Source: CAD feature listing. Evaluate the final solid. Frame: model axes, mm. Round coordinates to 2 decimals unless told otherwise and drop trailing zeros. Order: outer loops, then holes, each group sorted by start corner. A loop starts at its lowest first (then second) coordinate and runs counter-clockwise, first axis right, second up. Notation, with made-up numbers: M 14.25,58.5 L 19.25,58.5 A32 cw 19.25,92.5 Z; hole C 9,69 d2. An arc over 180 degrees is marked long. Answer in a Markdown table with one row per item. Add a question column.
```python
from build123d import *

# Parameters (mm, degrees)
F0_W     = 20
F0_H     = 20
F1_DEPTH = 25
F3_DEPTH = 20
F4_DEPTH = 30
F5_DEPTH = 25


with BuildPart() as f1:
    # F0 (on Front) → F1 (new body, symmetric)
    with BuildSketch(Plane.XZ):
        Rectangle(F0_W, F0_H)
        Polygon((20, -10), (10, 10), (10, -10), align=None)
        Polygon((20, 10), (10, 10), (20, -10), align=None)
        Polygon((-10, -10), (-10, 10), (-20, -10), align=None)
        Polygon((-20, -10), (-10, 10), (-20, 10), align=None)
    extrude(amount=F1_DEPTH, both=True)

    # F2 (on Right) → F3 (join, symmetric)
    with BuildSketch(Plane.YZ):
        Polygon((-25, -10), (-25, 0), (-25, 10), (-27.5, -10), align=None)
        Polygon((25, 10), (25, 0), (25, -10), (27.5, -10), align=None)
    extrude(amount=F3_DEPTH, both=True)

    # F0 (on Front) → F4 (cut, symmetric)
    with BuildSketch(Plane.XZ):
        Polygon((20, 10), (10, 10), (20, -10), align=None)
        Polygon((-20, -10), (-10, 10), (-20, 10), align=None)
    extrude(amount=F4_DEPTH, both=True, mode=Mode.SUBTRACT)

    # F2 (on Right) → F5 (cut, symmetric)
    with BuildSketch(Plane.YZ):
        Polygon((12.5, 9), (12.5, 10), (12, 10), align=None)
        Polygon((12.5, 9), (13, 10), (12.5, 10), align=None)
        Polygon((-12.5, 10), (-13, 10), (-12.5, 9), align=None)
        Polygon((-12, 10), (-12.5, 10), (-12.5, 9), align=None)
    extrude(amount=F5_DEPTH, both=True, mode=Mode.SUBTRACT)


solid = f1.part
```
(1) Draft query along Z for faces 1 (the face through (0, 0, 10)), 2 (the face through (0, 0, -10)). Return one class per face: +Z half, -Z half, draft (parallel to the pull), parting line (faces both ways), or undercut.
(2) Cut plane B-B (z = 6). Return loops of the section in (x, y), and give its area (3 significant figures).
(3) Cut plane A-A (x = 2). Return loops of the section in (y, z).
(4) Line query: line 1 (Z direction, x = 16, y = -14); line 2 (X direction, y = -2, z = -5.75) (3 decimals); line 3 (X direction, y = 19, z = 1.75) (3 decimals). Output: solid intervals per line, ascending. Write a range as from..to.
(5) Cut plane C-C (y = 1). Return loops of the section in (x, z), and give its area (3 significant figures).
(6) Pin query (flat end, axial travel): pin 1 (10 mm diameter, centred on x = 0, z = -1, fed in from +Y); pin 2 (3 mm diameter, centred on x = -6.5, z = -5, fed in from -Y); pin 3 (3 mm diameter, centred on y = -1, z = -7, fed in from -X). Return the tip coordinate at first contact, or that it passes through.
Answer list:
| question | item | result |
|---|---|---|
| 1 | face 1 | +Z half |
| 1 | face 2 | -Z half |
| 2 | outline | M -12,-25.5 L 12,-25.5 L 12,25.5 L -12,25.5 Z |
| 2 | area | 1,220 mm² |
| 3 | outline | M -27.5,-10 L 27.5,-10 L 25,10 L 13,10 L 12.5,9 L 12,10 L -12,10 L -12.5,9 L -13,10 L -25,10 Z |
| 4 | line 1 | -10..-2 |
| 4 | line 2 | -17.875..17.875 |
| 4 | line 3 | -14.125..14.125 |
| 5 | outline | M -20,-10 L 20,-10 L 10,10 L -10,10 Z |
| 5 | area | 600 mm² |
| 6 | pin 1 | y = 27 |
| 6 | pin 2 | y = -27.06 |
| 6 | pin 3 | x = -19.25 |
